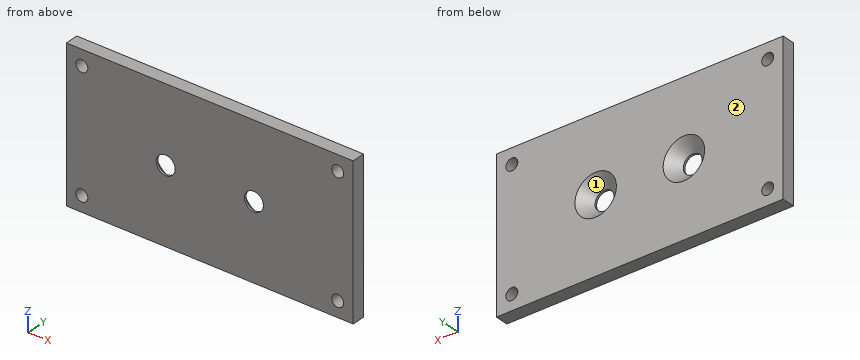
```python
from build123d import *

# Parameters (mm, degrees)
SKETCH1_W              = 65
SKETCH1_H              = 34
SKETCH1_R              = 0.5
BOSS_EXTRUDE1_DEPTH    = 3
M2_5_CLEARANCE_HOLE1_D = 2.7


# Read off the part's stored shape, not the designer's step: CSK for M4 Flat Head Machine Screw1
with BuildPart() as part:
    # Sketch1 → Boss-Extrude1 (new body)
    with BuildSketch(Plane(origin=(0, 0, 0), x_dir=(1, 0, 0), z_dir=(0, 1, 0))):
        Rectangle(SKETCH1_W, SKETCH1_H)
        with Locations(Location((-29, -13.5, 0), (0, 0, 270))):
            Circle(SKETCH1_R, mode=Mode.SUBTRACT)
        with Locations(Location((-29, 13.5, 0), (0, 0, 270))):
            Circle(SKETCH1_R, mode=Mode.SUBTRACT)
        with Locations(Location((29, -13.5, 0), (0, 0, 270))):
            Circle(SKETCH1_R, mode=Mode.SUBTRACT)
        with Locations(Location((29, 13.5, 0), (0, 0, 270))):
            Circle(SKETCH1_R, mode=Mode.SUBTRACT)
        with Locations(Location((-10, 0, 0), (0, 0, 270))):
            Circle(SKETCH1_R, mode=Mode.SUBTRACT)
        with Locations(Location((10, 0, 0), (0, 0, 270))):
            Circle(SKETCH1_R, mode=Mode.SUBTRACT)
    extrude(amount=BOSS_EXTRUDE1_DEPTH)

    # M2.5 Clearance Hole1 (through all)
    with Locations(Plane(origin=(0, 3, 0), x_dir=(1, 0, 0), z_dir=(0, 1, 0))):
        with Locations((-29, -13.5), (-29, 13.5), (29, 13.5), (29, -13.5)):
            Hole(M2_5_CLEARANCE_HOLE1_D / 2)

    # CSK for M4 Flat Head Machine Screw1 outl → CSK for M4 Flat Head Machine Screw1 (revolve, cut)
    with BuildSketch(Plane(origin=(10, 0, 0), x_dir=(1, 0, 0), z_dir=(0, 0, 1))):
        Polygon((0.5, 0), (2.15, 0), (2.15, 0.45), (4.7, 3), (0.5, 3), align=None)
    revolve(axis=Axis((10, 0, 0), (0, 1, 0)), mode=Mode.SUBTRACT)

    # CSK for M4 Flat Head Machine Screw1 2 ou → CSK for M4 Flat Head Machine Screw1 2 (revolve, cut)
    with BuildSketch(Plane(origin=(-10, 0, 0), x_dir=(1, 0, 0), z_dir=(0, 0, 1))):
        Polygon((0.5, 0), (2.15, 0), (2.15, 0.45), (4.7, 3), (0.5, 3), align=None)
    revolve(axis=Axis((-10, 0, 0), (0, 1, 0)), mode=Mode.SUBTRACT)


solid = part.part
```
Can you work these out from the model? Positions are in its coordinate system, mm. Face numbers are marked on the shaded views. Coordinates: 2 decimals unless noted, no trailing zeros. Write each loop counter-clockwise with the first axis right and the second up, starting at its lowest first coordinate (ties: lowest second). Pieces come first, ordered by that corner, then holes. Notation, with made-up numbers: (3.25, -27) - (56.25, -27) arc R8 ccw to (56.25, -23) - close; hole circle Ø5 at (87.5, 26). An arc over 180 degrees is marked (long way). Return JSON: item names as keys, results as strings.
Q1. If we section it at D-D (z = 0): Please give me the cut outline in (x, y).
Computed values:
{"outline": "(-32.5, 0) - (-12.15, 0) - (-12.15, 0.45) - (-14.7, 3) - (-32.5, 3) - close; (-7.85, 0) - (7.85, 0) - (7.85, 0.45) - (5.3, 3) - (-5.3, 3) - (-7.85, 0.45) - close; (12.15, 0) - (32.5, 0) - (32.5, 3) - (14.7, 3) - (12.15, 0.45) - close"}
Q2. Thinking about a two-plate mould opening in Z: for the marked faces 1 and 2, which applies, +Z half, -Z half, draft (parallel to the pull), parting line (faces both ways), or undercut?
Computed values:
{"face 1": "undercut", "face 2": "draft"}
Q3. If we section it at A-A (x = -10): Please give me the cut outline in (y, z).
Computed values:
{"outline": "(0, -17) - (3, -17) - (3, -4.7) - (0.45, -2.15) - (0, -2.15) - close; (0, 2.15) - (0.45, 2.15) - (3, 4.7) - (3, 17) - (0, 17) - close"}
Q4. Please list where these lines run through material, in increasing order: L1, parallel to Z at x = 29, y = 2.15; L2, parallel to X at y = 1, z = -13.5; L3, parallel to X at y = 2, z = 2.5. Write a range as from..to.
Computed values:
{"L1": "z = -17..-14.85, -12.15..12.15, 14.85..17", "L2": "x = -32.5..-30.35, -27.65..27.65, 30.35..32.5", "L3": "x = -32.5..-12.73, -7.27..7.27, 12.73..32.5"}
Q5. If we section it at B-B (z = 13.5): Please give me the cut outline in (x, y).
Computed values:
{"outline": "(-32.5, 0) - (-30.35, 0) - (-30.35, 3) - (-32.5, 3) - close; (-27.65, 0) - (27.65, 0) - (27.65, 3) - (-27.65, 3) - close; (30.35, 0) - (32.5, 0) - (32.5, 3) - (30.35, 3) - close"}
Q6. If we section it at C-C (x = -29): Please give me the cut outline in (y, z), then the cut area to 3 significant figures.
Computed values:
{"outline": "(0, -17) - (3, -17) - (3, -14.85) - (0, -14.85) - close; (0, -12.15) - (3, -12.15) - (3, 12.15) - (0, 12.15) - close; (0, 14.85) - (3, 14.85) - (3, 17) - (0, 17) - close", "area": "85.8 mm2"}
